```python
from build123d import *

# Parameters (mm, degrees)
CROQUIS2_R              = 2.75
SALIENTE_EXTRUIR1_DEPTH = 6
SALIENTE_EXTRUIR2_START = -6
SALIENTE_EXTRUIR2_DEPTH = 6
CORTAR_EXTRUIR1_DEPTH   = 71.114192572
CROQUIS5_R              = 1.5
CORTAR_EXTRUIR2_DEPTH   = 71.046461519


with BuildPart() as part:
    # Croquis2 → Saliente-Extruir1 (new body)
    with BuildSketch(Plane.XY):
        with BuildLine():
            Line((0, 0), (42.930999161, 0))
            Line((42.930999161, 0), (56.636539912, 15.69811875))
            ThreePointArc((56.636539912, 15.69811875), (56.30188125, 20.636539912), (51.363460088, 20.30188125))
            Line((51.363460088, 20.30188125), (39.75, 7))
            Line((39.75, 7), (31.75, 7))
            Line((31.75, 7), (31.75, 13))
            ThreePointArc((31.75, 13), (28, 16.75), (24.25, 13))
            Line((24.25, 13), (24.25, 7))
            Line((24.25, 7), (9.75, 7))
            Line((9.75, 7), (9.75, 13))
            ThreePointArc((9.75, 13), (6, 16.75), (2.25, 13))
            Line((2.25, 13), (2.25, 7))
            Line((2.25, 7), (0, 7))
            ThreePointArc((0, 7), (-3.5, 3.5), (0, 0))
        make_face()
        with Locations(Location((6, 13, 0), (0, 0, 180))):
            Circle(CROQUIS2_R, mode=Mode.SUBTRACT)
        with Locations(Location((28, 13, 0), (0, 0, 180))):
            Circle(CROQUIS2_R, mode=Mode.SUBTRACT)
    extrude(amount=SALIENTE_EXTRUIR1_DEPTH)

    # Croquis3 → Saliente-Extruir2 (add)
    with BuildSketch(Plane.XY.offset(6).offset(SALIENTE_EXTRUIR2_START)):
        with BuildLine():
            Line((51.363460088, 20.30188125), (46.467028822, 24.576803572))
            ThreePointArc((46.467028822, 24.576803572), (60.576803572, 25.532971178), (61.532971178, 11.423196428))
            Line((61.532971178, 11.423196428), (56.636539912, 15.69811875))
            ThreePointArc((56.636539912, 15.69811875), (56.30188125, 20.636539912), (51.363460088, 20.30188125))
        make_face()
    extrude(amount=SALIENTE_EXTRUIR2_DEPTH)

    # Croquis4 → Cortar-Extruir1 (cut, through all)
    with BuildSketch(Plane.XY.offset(6)):
        with BuildLine():
            ThreePointArc((49.70655821, 27.031409502), (47.593627222, 25.678436548), (45.883978244, 23.842105002))
            ThreePointArc((45.883978244, 23.842105002), (46.836617605, 23.831529671), (47.722398468, 23.480779257))
            ThreePointArc((47.722398468, 23.480779257), (48.610097364, 22.792823599), (49.70436623, 22.540102483))
            ThreePointArc((49.70436623, 22.540102483), (49.995888886, 22.799176411), (50.303002079, 23.03956411))
            ThreePointArc((50.303002079, 23.03956411), (50.250428059, 24.161405581), (49.732651549, 25.157999682))
            ThreePointArc((49.732651549, 25.157999682), (49.54628016, 26.09229048), (49.70655821, 27.031409502))
        make_face()
        with BuildLine():
            ThreePointArc((55.83506194, 27.830185536), (53.330407314, 27.977557098), (50.867903635, 27.496840125))
            ThreePointArc((50.867903635, 27.496840125), (51.632389044, 26.928337135), (52.142834895, 26.123925161))
            ThreePointArc((52.142834895, 26.123925161), (52.456628197, 25.045581024), (53.193364562, 24.197930244))
            ThreePointArc((53.193364562, 24.197930244), (53.581491179, 24.236172737), (53.971247316, 24.250133864))
            ThreePointArc((53.971247316, 24.250133864), (54.588115912, 25.188624914), (54.755009231, 26.299227874))
            ThreePointArc((54.755009231, 26.299227874), (55.153393963, 27.164631362), (55.83506194, 27.830185536))
        make_face()
        with BuildLine():
            ThreePointArc((61.262634381, 24.874164811), (59.322949053, 26.46558996), (57.048183382, 27.524105106))
            ThreePointArc((57.048183382, 27.524105106), (57.332507396, 26.614823277), (57.272645269, 25.664007776))
            ThreePointArc((57.272645269, 25.664007776), (56.892674603, 24.607165968), (56.990470215, 23.488359312))
            ThreePointArc((56.990470215, 23.488359312), (57.326949617, 23.291163037), (57.6504751, 23.073364917))
            ThreePointArc((57.6504751, 23.073364917), (58.701163476, 23.470033862), (59.488979049, 24.270433099))
            ThreePointArc((59.488979049, 24.270433099), (60.319950474, 24.736394558), (61.262634381, 24.874164811))
        make_face()
        with BuildLine():
            ThreePointArc((63.916127336, 19.292446773), (63.282305175, 21.720055193), (62.064160681, 23.913485649))
            ThreePointArc((62.064160681, 23.913485649), (61.75972119, 23.010739734), (61.152416384, 22.276699911))
            ThreePointArc((61.152416384, 22.276699911), (60.223817628, 21.645038081), (59.645317888, 20.682421665))
            ThreePointArc((59.645317888, 20.682421665), (59.80162638, 20.325108897), (59.935345471, 19.958743009))
            ThreePointArc((59.935345471, 19.958743009), (61.018526379, 19.662075794), (62.126345433, 19.846546004))
            ThreePointArc((62.126345433, 19.846546004), (63.072500712, 19.735083994), (63.916127336, 19.292446773))
        make_face()
        with BuildLine():
            ThreePointArc((62.781996685, 13.217057996), (63.696136214, 15.553585782), (63.99990269, 18.044115666))
            ThreePointArc((63.99990269, 18.044115666), (63.222985233, 17.492723921), (62.300207541, 17.255838039))
            ThreePointArc((62.300207541, 17.255838039), (61.177673859, 17.290629538), (60.143846005, 16.851890114))
            ThreePointArc((60.143846005, 16.851890114), (60.060279056, 16.470942186), (59.953115608, 16.095947847))
            ThreePointArc((59.953115608, 16.095947847), (60.655050756, 15.219261265), (61.659724067, 14.717341097))
            ThreePointArc((61.659724067, 14.717341097), (62.359664041, 14.071030318), (62.781996685, 13.217057996))
        make_face()
        with BuildLine():
            ThreePointArc((58.29344179, 8.968590498), (60.406372778, 10.321563452), (62.116021756, 12.157894998))
            ThreePointArc((62.116021756, 12.157894998), (61.163382395, 12.168470329), (60.277601532, 12.519220743))
            ThreePointArc((60.277601532, 12.519220743), (59.389902636, 13.207176401), (58.29563377, 13.459897517))
            ThreePointArc((58.29563377, 13.459897517), (58.004111114, 13.200823589), (57.696997921, 12.96043589))
            ThreePointArc((57.696997921, 12.96043589), (57.749571941, 11.838594419), (58.267348451, 10.842000318))
            ThreePointArc((58.267348451, 10.842000318), (58.45371984, 9.90770952), (58.29344179, 8.968590498))
        make_face()
    extrude(amount=-CORTAR_EXTRUIR1_DEPTH, mode=Mode.SUBTRACT)

    # Croquis5 → Cortar-Extruir2 (cut, through all)
    with BuildSketch(Plane.XY.offset(6)):
        with Locations((54, 18)):
            Circle(CROQUIS5_R)
    extrude(amount=-CORTAR_EXTRUIR2_DEPTH, mode=Mode.SUBTRACT)


solid = part.part
```
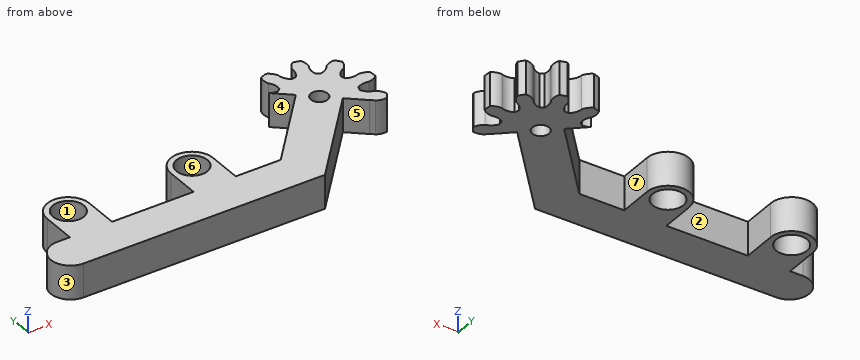
Work out the finished part from the listing and answer in its coordinate system (mm). Face numbers are marked on the shaded views. A direction names the side the tool comes from. Give positions to 0.01 mm unless a question says otherwise; leave off trailing zeros. Write each loop counter-clockwise with the first axis right and the second up, starting at its lowest first coordinate (ties: lowest second). Pieces come first, ordered by that corner, then holes. Notation, with made-up numbers: (23.5, 80.5) - (41.5, 80.5) arc R33 cw to (41.5, 114.5) - close; hole circle Ø4 at (70.5, -10). An arc over 180 degrees is marked (long way). Use one line per item in the form item = value.
1. Each of these flat-tipped pins is pushed along its axis until it touches: pin 1 Ø0.7 at (x, z) = (1.5, 2) entering from +Y; pin 2 Ø3 at (y, z) = (9, 4.5) entering from -X; pin 3 Ø1.5 at (x, z) = (55, 3) entering from -Y; pin 4 Ø2.5 at (x, y) = (54, 18) entering from +Z. Where does it stop, or does it pass through?
Filled in:
pin_1 = 7
pin_2 = 2.25
pin_3 = 12.96
pin_4 = through
2. A cutting plane is placed at B-B (y = 3.5). Write down the section's boundary in (x, z), and give its area (3 significant figures).
Filled in:
outline = (-3.5, 0) - (45.99, 0) - (45.99, 6) - (-3.5, 6) - close
area = 297 mm^2
3. A cutting plane is placed at A-A (x = 28). Write down the section's boundary in (y, z).
Filled in:
outline = (0, 0) - (10.25, 0) - (10.25, 6) - (0, 6) - close; (15.75, 0) - (16.75, 0) - (16.75, 6) - (15.75, 6) - close
4. A cutting plane is placed at C-C (z = 3.2). State how many separate pieces and enclosed holes the cut face has, and give its area (3 significant figures).
Filled in:
separate_pieces = 1
enclosed_holes = 3
area = 629 mm^2
5. Determine the mould class of the marked faces 1, 2, 3 and 4 for opening direction Y: released by +Y, released by -Y, zero draft, split by the parting line, or undercut.
Filled in:
face_1 = undercut
face_2 = released by +Y
face_3 = split by the parting line
face_4 = undercut
6. Consider L1, parallel to X at y = 9.25, z = 4.5; L2, parallel to X at y = 13, z = 4.65; L3, parallel to X at y = 9.75, z = 3.55. Determine where each line is inside the solid, lowest interval first.
Filled in:
L1 = 2.25 to 9.75, 24.25 to 31.75, 41.71 to 51.01
L2 = 2.25 to 3.25, 8.75 to 9.75, 24.25 to 25.25, 30.75 to 31.75, 44.99 to 54.28, 59.75 to 62.66
L3 = 2.25 to 9.75, 24.25 to 31.75, 42.15 to 51.44
7. For the marked faces 5, 6 and 7, determine the directions among +Z, -Z, +X, -X, +Y, -Y from which every point of the face is accessible in a straight line to the end or side of a thin tool.
Filled in:
face_5 = +Z, -Z, -Y
face_6 = +Z, -Z
face_7 = +Z, -Z, +Y
